Could you check a few things on this model? Use its own coordinates, in mm. Face numbers are marked on the shaded views. Give positions to 0.01 mm unless a question says otherwise; leave off trailing zeros. Order: outer loops, then holes, each group sorted by start corner. A loop starts at its lowest first (then second) coordinate and runs counter-clockwise, first axis right, second up. Notation, with made-up numbers: M 55,19.5 L 80,19.5 A7 cw 80,31.5 Z; hole C 79.25,77 d10. An arc over 180 degrees is marked long. Return JSON: item names as keys, results as strings. Group by question number.
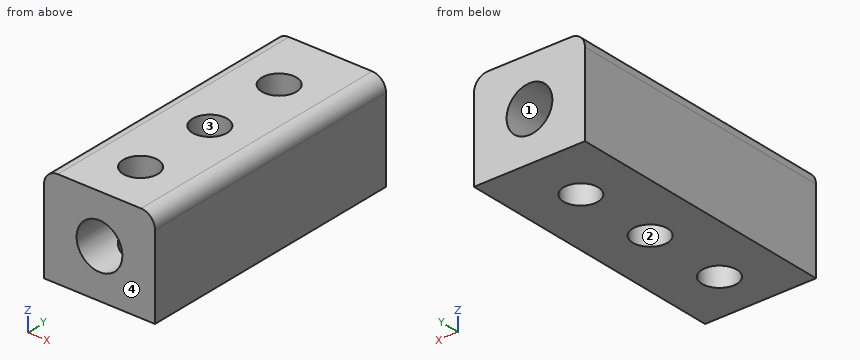
```python
from build123d import *

# Parameters (mm, degrees)
F0_W     = 8
F0_H     = 7
F0_R     = 1.65
F1_DEPTH = 20
F2_R     = 1.25
F3_DEPTH = 7.001
F4_R     = 1


with BuildPart() as f1:
    # F0 (on Front) → F1 (new body)
    with BuildSketch(Plane.XZ):
        Rectangle(F0_W, F0_H)
        Circle(F0_R, mode=Mode.SUBTRACT)
    extrude(amount=-F1_DEPTH)

    # F2 (on face) → F3 (cut, through all)
    with BuildSketch(Plane.XY.offset(3.5)):
        with Locations((0, 15.555)):
            Circle(F2_R)
        with Locations((0, 9.555)):
            Circle(F2_R)
        with Locations((0, 3.555)):
            Circle(F2_R)
    extrude(amount=-F3_DEPTH, mode=Mode.SUBTRACT)

    # F4
    f4_edges = [f1.edges().sort_by_distance(p)[0] for p in [
        (4, 10, 3.5),
        (-4, 10, 3.5),
    ]]
    fillet(f4_edges, radius=F4_R)


solid = f1.part
```
1. If we mould it in two halves opening along Y, with no side actions, what happens to the marked faces 1, 2, 3 and 4? For each: pulls with the +Y half, pulls with the -Y half, needs draft (parallel to the pull), parting line crosses it, or undercut.
2. Imagine slicing it at D-D, the plane y = 12. Please give me the cut outline in (x, z).
3. I need wall thicknesses on L1, parallel to Y at x = 0, z = 2 (3 decimals); L2, parallel to Y at x = 1, z = 3.25 (3 decimals); L3, parallel to X at y = 8.5, z = -1.25. Which ranges of each line are inside material? Lowest first, please. Write a range as from..to.
4. Imagine slicing it at A-A, the plane x = 0. Count the separate pieces of the cut face and the enclosed holes in it, plus the area to 4 significant figures.
5. Imagine slicing it at B-B, the plane z = 0. Please give me the cut outline in (x, y).
6. Imagine slicing it at C-C, the plane y = 9. Please give me the cut outline in (x, z), plus the area to 3 significant figures.
Values:
{
 "1": {"face 1": "needs draft", "face 2": "undercut", "face 3": "undercut", "face 4": "pulls with the -Y half"},
 "2": {"outline": "M -4,-3.5 L 4,-3.5 L 4,2.5 A1 ccw 3,3.5 L -3,3.5 A1 ccw -4,2.5 Z; hole C 0,0 d3.3"},
 "3": {"L1": "y = 0..2.305, 4.805..8.305, 10.805..14.305, 16.805..20", "L2": "y = 0..2.805, 4.305..8.805, 10.305..14.805, 16.305..20", "L3": "x = -4..-1.08, 1.08..4"},
 "4": {"separate pieces": "8", "enclosed holes": "0", "area": "46.25 mm²"},
 "5": {"outline": "M -4,0 L -1.65,0 L -1.65,20 L -4,20 Z; M 1.65,0 L 4,0 L 4,20 L 1.65,20 Z"},
 "6": {"outline": "M -4,-3.5 L -1.12,-3.5 L -1.12,-1.21 A1.65 cw -1.12,1.21 L -1.12,3.5 L -3,3.5 A1 ccw -4,2.5 Z; M 1.12,-3.5 L 4,-3.5 L 4,2.5 A1 ccw 3,3.5 L 1.12,3.5 L 1.12,1.21 A1.65 cw 1.12,-1.21 Z", "area": "38.1 mm²"}
}
